```python
from build123d import *

# Parameters (mm, degrees)
SKETCH1_R           = 1
BOSS_EXTRUDE1_DEPTH = 5


with BuildPart() as part:
    # Sketch1 → Boss-Extrude1 (new body)
    with BuildSketch(Plane(origin=(0, 0, 0), x_dir=(1, 0, 0), z_dir=(0, 1, 0))):
        with BuildLine():
            Line((0, 75), (0, 53.165914195))
            ThreePointArc((0, 53.165914195), (4.315565807, 44.938690611), (13.537441581, 43.812491984))
            ThreePointArc((13.537441581, 43.812491984), (80.9029452, 45.023033848), (133.74584981, 3.223465408))
            ThreePointArc((133.74584981, 3.223465408), (133.255689752, 0.004881448), (130, 0))
            ThreePointArc((130, 0), (65, 24.006579232), (0, 0))
            Line((0, 0), (-15, 0))
            Line((-15, 0), (-15, 75))
            Line((-15, 75), (0, 75))
        make_face()
        with Locations(Location((-7.5, 10, 0), (0, 0, 270))):
            Circle(SKETCH1_R, mode=Mode.SUBTRACT)
        with Locations(Location((-7.5, 20, 0), (0, 0, 270))):
            Circle(SKETCH1_R, mode=Mode.SUBTRACT)
        with Locations(Location((-7.5, 65, 0), (0, 0, 270))):
            Circle(SKETCH1_R, mode=Mode.SUBTRACT)
        with Locations(Location((85, 27.5, 0), (0, 0, 270))):
            Circle(SKETCH1_R, mode=Mode.SUBTRACT)
        with Locations(Location((45, 35, 0), (0, 0, 270))):
            Circle(SKETCH1_R, mode=Mode.SUBTRACT)
    extrude(amount=BOSS_EXTRUDE1_DEPTH)


solid = part.part
```
CAD build for the part. Positions are in the model's coordinates, mm. A direction names the side the tool comes from. Round coordinates to 2 decimals unless told otherwise and drop trailing zeros. Loops run counter-clockwise (first coordinate to the right, second up) from the corner with the lowest first, then second, coordinate; pieces in that order, holes last. Notation, with made-up numbers: M 71,17 L 93,17 A36 ccw 93,52 Z; hole C -3.5,35.5 d11. An arc over 180 degrees is marked long. Return JSON: item names as keys, results as strings. Group by question number.
(1) Wall check: probe 1 along X at (y, z) = (1.3, -10); probe 2 along X at (y, z) = (2.6, -70); probe 3 along Z at (x, y) = (85, 2.9). Give the ranges that are in metal, low to high. Write a range as [from, to].
(2) Saw through at A-A, the plane z = -13.5. List the corners of the cut face in (x, y).
(3) Saw through at C-C, the plane z = -59.5. List the corners of the cut face in (x, y), and give its area (3 significant figures).
(4) Saw through at D-D, the plane x = 67. List the corners of the cut face in (y, z), and give its area (3 significant figures).
(5) Mould opens along X. For faces 3 (the flat face through (-15, 2, -37)), 4 (the flat face through (0, 2, -64)), 5 (the flat face through (44, 0, -29)), 6 (the cylindrical face through (79.99, 2.465, -45.326)) say: +X half, -X half, draft (parallel to the pull), parting line (faces both ways), or undercut.
(6) Tool access for faces 1 (the flat face through (-8, 2, -75)), 2 (the flat face through (-7, 2, 0)): list every direction of +Z, -Z, +X, -X, +Y, -Y with a clear straight run to the whole face (end or side of a thin tool).
(7) Drop flat-ended pins along their axis: P1, Ø2, axis at x = 10.5, y = 1.5, coming from the +Z side; P2, Ø2.5, axis at x = -7.5, z = -10, coming from the -Y side; P3, Ø1, axis at x = 67, y = 1.5, coming from the -Z side. Give the stop position or say it passes through.
(8) Saw through at B-B, the plane y = 2.8. List the corners of the cut face in (x, z) (1 decimal), and give its area (3 significant figures).
Answer list:
{
 "1": {"probe 1": "[-15, -8.5], [-6.5, 13.96], [116.04, 129.12]", "probe 2": "[-15, 0]", "probe 3": "[-43.54, -28.5], [-26.5, -21.99]"},
 "2": {"outline": "M -15,0 L 20.38,0 L 20.38,5 L -15,5 Z; M 109.62,0 L 126.39,0 L 126.39,5 L 109.62,5 Z"},
 "3": {"outline": "M -15,0 L 0,0 L 0,5 L -15,5 Z", "area": "75.0 mm2"},
 "4": {"outline": "M 0,-48.63 L 5,-48.63 L 5,-23.99 L 0,-23.99 Z", "area": "123 mm2"},
 "5": {"face 3": "-X half", "face 4": "+X half", "face 5": "draft", "face 6": "undercut"},
 "6": {"face 1": "-Z, +X, -X, +Y, -Y", "face 2": "+Z, -X, +Y, -Y"},
 "7": {"P1": "z = -7.19", "P2": "y = 0", "P3": "z = -48.72"},
 "8": {"outline": "M -15,-75 L 0,-75 L 0,-53.2 A10 cw 13.5,-43.8 A100 ccw 133.7,-3.2 A2.5 ccw 130,0 A100 cw 0,0 L -15,0 Z; hole C -7.5,-65 d2; hole C -7.5,-20 d2; hole C -7.5,-10 d2; hole C 45,-35 d2; hole C 85,-27.5 d2", "area": "4,380 mm2"}
}
